Part model, mm, in its own coordinate system. Face numbers are marked on the shaded views. A direction names the side the tool comes from. Round coordinates to 2 decimals unless told otherwise and drop trailing zeros. Order: outer loops, then holes, each group sorted by start corner. A loop starts at its lowest first (then second) coordinate and runs counter-clockwise, first axis right, second up. Notation, with made-up numbers: (62, 24.25) -> (95, 24.25) arc R8 cw to (95, 34.25) -> close; hole circle Ø9 at (76, 11). An arc over 180 degrees is marked (long way). Return JSON: item names as keys, results as strings. Group by question number.
Autodesk Inventor part; units mm, degrees
ref_plane "YZ Plane" through (0, 0, 0) normal (1, 0, 0) x (0, 1, 0)
ref_plane "XZ Plane" through (0, 0, 0) normal (0, 1, 0) x (-1, 0, 0)
ref_plane "XY Plane" through (0, 0, 0) normal (0, 0, 1) x (1, 0, 0)
sketch "Boceto1" plane through (0, 0, 0) normal (0, 1, 0) x (-1, 0, 0)
  line L0 (0, 0) -> (23, 0)
  line L1 (23, 0) -> (23, -43.3)
  line L2 (23, -43.3) -> (0, -43.3)
  line L3 (0, -43.3) -> (0, 0)
  dimension "d0" = 23
  dimension "d1" = 43.3
ref_plane "Plano de trabajo1" through (0, 92, 0) normal (0, 1, 0) x (1, 0, 0)
sketch "Boceto2" plane through (0, 92, 0) normal (0, 1, 0) x (1, 0, 0)
  line L0 (0, 43.3) -> (-23, 43.3)
  line L1 (-23, 43.3) -> (-23, 0)
  line L2 (-23, 0) -> (0, 0)
  line L3 (0, 0) -> (0, 43.3)
  line L4 (-26, -1) -> (-26, 44.3)
  line L5 (-24, 46.3) -> (1, 46.3)
  line L6 (3, 44.3) -> (3, -1)
  line L7 (1, -3) -> (-24, -3)
  arc A0 (-26, -1) -> (-24, -3) centre (-24, -1) ccw
  arc A1 (1, -3) -> (3, -1) centre (1, -1) ccw
  arc A2 (3, 44.3) -> (1, 46.3) centre (1, 44.3) ccw
  arc A3 (-24, 46.3) -> (-26, 44.3) centre (-24, 44.3) ccw
  point P0 (-11.5, 21.65)
  point P1 (-26, -3)
  point P2 (-26, 46.3)
  point P3 (3, 46.3)
  point P4 (3, -3)
  dimension "d4" = 21.65
  dimension "d5" = 11.5
  dimension "d6" = 3
  dimension "d9" = 2
extrude "Extrusión2" add sketch "Boceto2" against normal blind 92
sketch "Boceto3" plane through (0, 0, 0) normal (0, -1, 0) x (1, 0, 0)
  line L0 (3, -44.3) -> (3, 1)
  arc A0 (3, 1) -> (1, 3) centre (1, 1) ccw
  line L1 (1, 3) -> (-24, 3)
  arc A1 (-24, 3) -> (-26, 1) centre (-24, 1) ccw
  line L2 (-26, 1) -> (-26, -44.3)
  arc A2 (-26, -44.3) -> (-24, -46.3) centre (-24, -44.3) ccw
  line L3 (-24, -46.3) -> (1, -46.3)
  arc A3 (1, -46.3) -> (3, -44.3) centre (1, -44.3) ccw
  point P0 (0, 0)
extrude "Extrusión3" add sketch "Boceto3" along normal blind 3
sketch "Boceto4" plane through (0, -3, 0) normal (0, -1, 0) x (1, 0, 0)
  line L0 (3, -44.3) -> (3, 1)
  line L1 (3, -8.65) -> (5.8, -8.65)
  line L2 (5.8, -8.65) -> (5.8, -11.55)
  line L3 (5.8, -11.55) -> (8.7, -11.55)
  line L4 (8.7, -11.55) -> (8.7, -5.65)
  line L5 (8.7, -5.65) -> (3, -5.65)
  line L6 (3, -21.65) -> (22.5352, -21.65) construction
  line L7 (3, -34.65) -> (5.8, -34.65)
  line L8 (5.8, -34.65) -> (5.8, -31.75)
  line L9 (5.8, -31.75) -> (8.7, -31.75)
  line L10 (8.7, -31.75) -> (8.7, -37.65)
  line L11 (8.7, -37.65) -> (3, -37.65)
  point P0 (0, 0)
  point P1 (3, -37.65)
  dimension "d12" = 2.8
  dimension "d13" = 2.9
  dimension "d14" = 2.9
  dimension "d15" = 5.9
  dimension "d16" = 13
extrude "Extrusión4" add sketch "Boceto4" against normal blind 37
sketch "Boceto5" plane through (0, -3, 0) normal (0, -1, 0) x (1, 0, 0)
  line L0 (3, -34.65) -> (3, -8.65)
  line L1 (3, -8.65) -> (5.8, -8.65)
  line L2 (5.8, -8.65) -> (5.8, -11.55)
  line L3 (5.8, -31.75) -> (5.8, -34.65)
  line L4 (5.8, -34.65) -> (3, -34.65)
  line L5 (5.8, -11.55) -> (8.7, -11.55)
  line L6 (8.7, -31.75) -> (5.8, -31.75)
  line L7 (8.7, -11.55) -> (8.7, -31.75)
  point P0 (0, 0)
extrude "Extrusión5" add sketch "Boceto5" against normal blind 3
sketch "Boceto6" plane through (0, -3, 0) normal (0, -1, 0) x (1, 0, 0)
  arc A0 (3, 1) -> (1, 3) centre (1, 1) ccw
  line L0 (1, 3) -> (-24, 3)
  arc A1 (-24, 3) -> (-26, 1) centre (-24, 1) ccw
  line L1 (-26, 1) -> (-26, -44.3)
  arc A2 (-26, -44.3) -> (-24, -46.3) centre (-24, -44.3) ccw
  line L2 (-24, -46.3) -> (1, -46.3)
  arc A3 (1, -46.3) -> (3, -44.3) centre (1, -44.3) ccw
  line L3 (3, -44.3) -> (3, -37.65)
  line L4 (3, -37.65) -> (8.7, -37.65)
  line L5 (8.7, -37.65) -> (8.7, -5.65)
  line L6 (8.7, -5.65) -> (3, -5.65)
  line L7 (3, -5.65) -> (3, 1)
  line L8 (0, -43.3) -> (-23, -43.3)
  line L9 (3, -8.65) -> (3, -34.65)
  point P0 (0, 0)
  point P1 (-11.5, -21.65)
  dimension "d21" = 21.65
  dimension "d22" = 14.5
hole "Agujero1" at (-11.5, -3, -21.65) direction (0, 1, 0) diameter 20 end through all
sketch "Boceto7" plane through (0, -3, 0) normal (0, -1, 0) x (1, 0, 0)
  line L0 (1, 3) -> (-24, 3)
  line L1 (-3.95, 3) -> (-3.95, 5.8)
  line L2 (-3.95, 5.8) -> (-6.85, 5.8)
  line L3 (-6.85, 5.8) -> (-6.85, 8.7)
  line L4 (-6.85, 8.7) -> (-0.95, 8.7)
  line L5 (-0.95, 8.7) -> (-0.95, 3)
  line L6 (-11.5, 3) -> (-11.5, 18.2857) construction
  line L7 (-19.05, 3) -> (-19.05, 5.8)
  line L8 (-19.05, 5.8) -> (-16.15, 5.8)
  line L9 (-16.15, 5.8) -> (-16.15, 8.7)
  line L10 (-16.15, 8.7) -> (-22.05, 8.7)
  line L11 (-22.05, 8.7) -> (-22.05, 3)
  line L12 (8.7, -11.55) -> (8.7, -31.75) construction
  line L13 (8.7, -21.65) -> (17.1818, -21.65) construction
  line L14 (1, -46.3) -> (-24, -46.3)
  line L15 (-3.95, -46.3) -> (-3.95, -49.1)
  line L16 (-3.95, -49.1) -> (-6.85, -49.1)
  line L17 (-6.85, -49.1) -> (-6.85, -52)
  line L18 (-6.85, -52) -> (-0.95, -52)
  line L19 (-0.95, -52) -> (-0.95, -46.3)
  line L20 (-16.15, -52) -> (-22.05, -52)
  line L21 (-16.15, -49.1) -> (-16.15, -52)
  line L22 (-19.05, -49.1) -> (-16.15, -49.1)
  line L23 (-19.05, -46.3) -> (-19.05, -49.1)
  line L24 (-22.05, -52) -> (-22.05, -46.3)
  point P0 (0, 0)
  dimension "d30" = 2.8
  dimension "d31" = 2.9
  dimension "d32" = 2.9
  dimension "d33" = 5.9
  dimension "d34" = 7.55
extrude "Extrusión6" add sketch "Boceto7" against normal blind 21
sketch "Boceto8" plane through (0, -3, 0) normal (0, -1, 0) x (1, 0, 0)
  circle A0 centre (-11.5, -21.65) radius 10
  arc A1 (3, 1) -> (1, 3) centre (1, 1) ccw
  line L0 (1, 3) -> (-0.95, 3)
  line L1 (-0.95, 3) -> (-0.95, 8.7)
  line L2 (-0.95, 8.7) -> (-6.85, 8.7)
  line L3 (-6.85, 8.7) -> (-6.85, 5.8)
  line L4 (-6.85, 5.8) -> (-3.95, 5.8)
  line L5 (-3.95, 5.8) -> (-3.95, 3)
  line L6 (-3.95, 3) -> (-19.05, 3)
  line L7 (-19.05, 3) -> (-19.05, 5.8)
  line L8 (-19.05, 5.8) -> (-16.15, 5.8)
  line L9 (-16.15, 5.8) -> (-16.15, 8.7)
  line L10 (-16.15, 8.7) -> (-22.05, 8.7)
  line L11 (-22.05, 8.7) -> (-22.05, 3)
  line L12 (-22.05, 3) -> (-24, 3)
  arc A2 (-24, 3) -> (-26, 1) centre (-24, 1) ccw
  line L13 (-26, 1) -> (-26, -44.3)
  arc A3 (-26, -44.3) -> (-24, -46.3) centre (-24, -44.3) ccw
  line L14 (-24, -46.3) -> (-22.05, -46.3)
  line L15 (-22.05, -46.3) -> (-22.05, -52)
  line L16 (-22.05, -52) -> (-16.15, -52)
  line L17 (-16.15, -52) -> (-16.15, -49.1)
  line L18 (-16.15, -49.1) -> (-19.05, -49.1)
  line L19 (-19.05, -49.1) -> (-19.05, -46.3)
  line L20 (-19.05, -46.3) -> (-3.95, -46.3)
  line L21 (-3.95, -46.3) -> (-3.95, -49.1)
  line L22 (-3.95, -49.1) -> (-6.85, -49.1)
  line L23 (-6.85, -49.1) -> (-6.85, -52)
  line L24 (-6.85, -52) -> (-0.95, -52)
  line L25 (-0.95, -52) -> (-0.95, -46.3)
  line L26 (-0.95, -46.3) -> (1, -46.3)
  arc A4 (1, -46.3) -> (3, -44.3) centre (1, -44.3) ccw
  line L27 (3, -44.3) -> (3, -37.65)
  line L28 (3, -37.65) -> (8.7, -37.65)
  line L29 (8.7, -37.65) -> (8.7, -5.65)
  line L30 (8.7, -5.65) -> (3, -5.65)
  line L31 (3, -5.65) -> (3, 1)
  line L32 (-6.85, 8.7) -> (-16.15, 8.7)
  line L33 (-6.85, -52) -> (-16.15, -52)
  point P0 (0, 0)
extrude "Extrusión7" add sketch "Boceto8" against normal blind 3 contours L3 L4 L5 L6 L7 L8 L9 L32
sketch "Boceto9" plane through (0, 92, 0) normal (0, 1, 0) x (1, 0, 0)
  line L0 (3, -1) -> (3, 44.3)
  arc A0 (3, 44.3) -> (1, 46.3) centre (1, 44.3) ccw
  line L1 (1, 46.3) -> (-24, 46.3)
  arc A1 (-24, 46.3) -> (-26, 44.3) centre (-24, 44.3) ccw
  line L2 (-26, 44.3) -> (-26, -1)
  arc A2 (-26, -1) -> (-24, -3) centre (-24, -1) ccw
  line L3 (-24, -3) -> (1, -3)
  arc A3 (1, -3) -> (3, -1) centre (1, -1) ccw
  line L4 (0, 43.3) -> (0, 0)
  line L5 (0, 0) -> (-23, 0)
  line L6 (-23, 0) -> (-23, 43.3)
  line L7 (-23, 43.3) -> (0, 43.3)
extrude "Extrusión8" add sketch "Boceto9" along normal blind 3
fillet "Empalme1" radius 1.5 4 edges at (-11.5, 95, 0) (0, 95, -21.65) (-23, 95, -21.65) (-11.5, 95, -43.3)
fillet "Empalme2" radius 1 8 edges at (2.4142, 95, 2.4142) (3, 95, -21.65) (2.4142, 95, -45.7142) (-11.5, 95, -46.3) (-25.4142, 95, -45.7142) (-26, 95, -21.65) (-25.4142, 95, 2.4142) (-11.5, 95, 3)
sketch "Boceto10" plane through (0, 18, 0) normal (0, 1, 0) x (1, 0, 0)
  line L0 (-0.95, 46.3) -> (-0.95, 52)
  line L1 (-0.95, 52) -> (-6.85, 52)
  line L2 (-6.85, 52) -> (-6.85, 49.1)
  line L3 (-6.85, 49.1) -> (-3.95, 49.1)
  line L4 (-3.95, 49.1) -> (-3.95, 46.3)
  line L5 (-0.95, 46.3) -> (-3.95, 46.3)
  line L6 (-16.15, 49.1) -> (-16.15, 52)
  line L7 (-16.15, 52) -> (-22.05, 52)
  line L8 (-22.05, 52) -> (-22.05, 46.3)
  line L9 (-19.05, 46.3) -> (-22.05, 46.3)
  line L10 (-19.05, 46.3) -> (-19.05, 49.1)
  line L11 (-19.05, 49.1) -> (-16.15, 49.1)
  point P0 (0, 0)
extrude "Extrusión9" add sketch "Boceto10" along normal blind 20
fillet "Empalme3" radius 1 12 edges at (8.7, 15.5, -37.65) (8.7, 15.5, -5.65) (-0.95, 7.5, 8.7) (-22.05, 7.5, 8.7) (5.85, 34, -37.65) (5.85, 34, -5.65) (-0.95, 18, 5.85) (-22.05, 18, 5.85) (-0.95, 17.5, -52) (-0.95, 38, -49.15) (-22.05, 17.5, -52) (-22.05, 38, -49.15)
properties part number "cajaPilas"
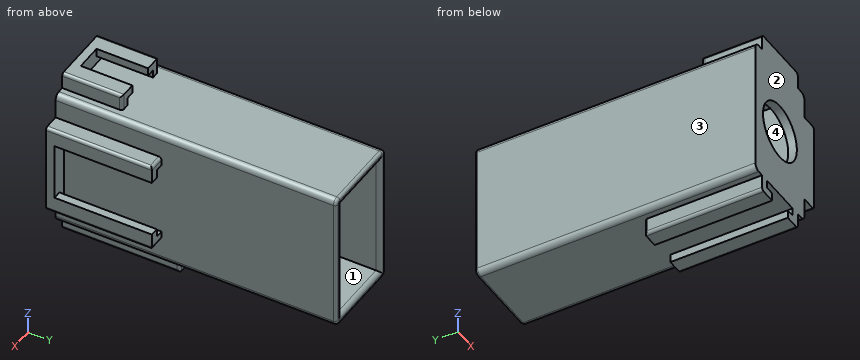
(1) Saw through at B-B, the plane z = -21.65. List the corners of the cut face in (x, y), and give its area (3 significant figures).
(2) Pin check, flat tips, straight feed: P1, Ø5, axis at x = -22, y = 64.5, coming from the +Z side; P2, Ø10, axis at x = -5.5, z = -20, coming from the +Y side; P3, Ø2.5, axis at x = -19, z = 6.5, coming from the +Y side. Stop position of each tip, or through.
(3) Tool access for the marked faces 3 and 4: list every direction of +Z, -Z, +X, -X, +Y, -Y with a clear straight run to the whole face (end or side of a thin tool).
(4) Saw through at A-A, the plane y = 60. List the corners of the cut face in (x, z), and give its area (3 significant figures).
(5) Probe L1, parallel to Z at x = -11.5, y = -2.2; L2, parallel to X at y = -1, z = -21; L3, parallel to X at y = 8, z = -22.5. List the from-to ranges inside material, lowest first. Write a range as [from, to].
(6) Mould opens along Z. For the marked faces 1 and 2 say: pulls with the +Z half, pulls with the -Z half, needs draft (parallel to the pull), parting line crosses it, or undercut.
(7) Saw through at C-C, the plane x = -11.5. List the corners of the cut face in (y, z).
(8) Saw through at D-D, the plane z = -39. List the corners of the cut face in (x, y), and give its area (3 significant figures).
Results are:
{
 "1": {"outline": "(-26, -3) -> (-21.5, -3) -> (-21.5, 0) -> (-23, 0) -> (-23, 93.5) arc R1.5 ccw to (-24.5, 95) -> (-25, 95) arc R1 ccw to (-26, 94) -> close; (-1.5, -3) -> (8.7, -3) -> (8.7, 0) -> (3, 0) -> (3, 94) arc R1 ccw to (2, 95) -> (1.5, 95) arc R1.5 ccw to (0, 93.5) -> (0, 0) -> (-1.5, 0) -> close", "area": "613 mm^2"},
 "2": {"P1": "stops at z = 3", "P2": "stops at y = 0", "P3": "stops at y = 18"},
 "3": {"face 3": "+Z, -Z, -X, +Y, -Y", "face 4": "+Y"},
 "4": {"outline": "(-26, -44.3) arc R2 ccw to (-24, -46.3) -> (1, -46.3) arc R2 ccw to (3, -44.3) -> (3, 1) arc R2 ccw to (1, 3) -> (-24, 3) arc R2 ccw to (-26, 1) -> close; hole (-23, -43.3) -> (0, -43.3) -> (0, 0) -> (-23, 0) -> close", "area": "430 mm^2"},
 "5": {"L1": "z = [-46.3, -31.65], [-11.65, 8.7]", "L2": "x = [-26, -21.48], [-1.52, 8.7]", "L3": "x = [-26, -23], [0, 3]"},
 "6": {"face 1": "undercut", "face 2": "needs draft"},
 "7": {"outline": "(-3, -46.3) -> (94, -46.3) arc R1 ccw to (95, -45.3) -> (95, -44.8) arc R1.5 ccw to (93.5, -43.3) -> (0, -43.3) -> (0, -31.65) -> (-3, -31.65) -> close; (-3, -11.65) -> (0, -11.65) -> (0, 0) -> (93.5, 0) arc R1.5 ccw to (95, 1.5) -> (95, 2) arc R1 ccw to (94, 3) -> (0, 3) -> (0, 8.7) -> (-3, 8.7) -> close"},
 "8": {"outline": "(-26, -3) -> (3, -3) -> (3, 94) arc R1 ccw to (2, 95) -> (1.5, 95) arc R1.5 ccw to (0, 93.5) -> (0, 0) -> (-23, 0) -> (-23, 93.5) arc R1.5 ccw to (-24.5, 95) -> (-25, 95) arc R1 ccw to (-26, 94) -> close", "area": "656 mm^2"}
}
